Input: part model. Units: mm. Frame: model coordinates. A direction names the side the tool comes from. Round coordinates to 2 decimals unless told otherwise and drop trailing zeros. Write each loop counter-clockwise with the first axis right and the second up, starting at its lowest first coordinate (ties: lowest second). Pieces come first, ordered by that corner, then holes. Notation, with made-up numbers: (61, 51.25) -> (110, 51.25) arc R15 ccw to (110, 80.25) -> close; hole circle Ø8 at (60.25, 47). An arc over 180 degrees is marked (long way). Use CSV: the item, a comma, the result in double quotes.
```python
from build123d import *

# Parameters (mm, degrees)
SKIZZE1_W                       = 10
SKIZZE1_H                       = 46.07297751
SKIZZE1_R                       = 1.75
SKIZZE1_W_2                     = 3.5
SKIZZE1_H_2                     = 13
AUFSATZ_LINEAR_AUSTRAGEN1_DEPTH = 5
SKIZZE2_W                       = 5
SKIZZE2_H                       = 5
SCHNITT_LINEAR_AUSTRAGEN2_DEPTH = 2


with BuildPart() as part:
    # Skizze1 → Aufsatz-Linear austragen1 (new body)
    # profile 1 of 5: a face of its own
    with BuildSketch(Plane.XY):
        with Locations((0, 10.889252833)):
            Rectangle(SKIZZE1_W, SKIZZE1_H)
        with Locations((0, -1.574258412)):
            Circle(SKIZZE1_R, mode=Mode.SUBTRACT)
        with Locations((0, 7.425741588)):
            Circle(SKIZZE1_R, mode=Mode.SUBTRACT)
    # profile 2 of 5: a face of its own
    with BuildSketch(Plane.XY):
        Polygon((10, 30.925741588), (5, 30.925741588), (5, 30.675741588), (5, 18.175741588), (5, 17.925741588), (10, 17.925741588), align=None)
    # profile 3 of 5: a face of its own
    with BuildSketch(Plane.XY):
        Polygon((33.5, 17.925741588), (10, 17.925741588), (5, 17.925741588), (5, 14.925741588), (37, 14.925741588), (37, 17.925741588), align=None)
    # profile 4 of 5: a face of its own
    with BuildSketch(Plane.XY):
        Polygon((37, 33.925741588), (5, 33.925741588), (5, 30.925741588), (10, 30.925741588), (33.5, 30.925741588), (37, 30.925741588), align=None)
    # profile 5 of 5: a face of its own
    with BuildSketch(Plane.XY):
        with Locations((35.25, 24.425741588)):
            Rectangle(SKIZZE1_W_2, SKIZZE1_H_2)
    extrude(amount=AUFSATZ_LINEAR_AUSTRAGEN1_DEPTH)

    # Skizze2 → Schnitt-Linear austragen2 (cut)
    with BuildSketch(Plane(origin=(0, 0, 5), x_dir=(-1, 0, 0), z_dir=(0, 0, -1))):
        with Locations((0, 22.425741588)):
            Rectangle(SKIZZE2_W, SKIZZE2_H)
    extrude(amount=SCHNITT_LINEAR_AUSTRAGEN2_DEPTH, mode=Mode.SUBTRACT)


solid = part.part
```
Item 1: Set-up query: faces 4 (the face through (11, 16, 5)), 5 (the face through (22, 17.926, 2)), 6 (the face through (0, 19.926, 4)), 7 (the face through (5, 1, 2)), 8 (the face through (11, 16, 0)). Return all of +Z, -Z, +X, -X, +Y, -Y with unobstructed straight access to the full face (end or side cutting, diameter ignored); none if empty.
Worked answers:
face 4,"+Z, +X, -X, +Y, -Y"
face 5,"+Z, -Z"
face 6,"+Z"
face 7,"+Z, -Z, +X, -Y"
face 8,"-Z, +X, -X, +Y, -Y"
Item 2: Section query B-B on x = 0. Return the cut outline in (y, z).
Worked answers:
outline,"(-12.15, 0) -> (-3.32, 0) -> (-3.32, 5) -> (-12.15, 5) -> close; (0.18, 0) -> (5.68, 0) -> (5.68, 5) -> (0.18, 5) -> close; (9.18, 0) -> (33.93, 0) -> (33.93, 5) -> (24.93, 5) -> (24.93, 3) -> (19.93, 3) -> (19.93, 5) -> (9.18, 5) -> close"
Item 3: First-contact query: pin 1 Ø2.5 at (x, z) = (20, 1.5) entering from -Y; pin 2 Ø3 at (x, y) = (0, 7.43) entering from +Z; pin 3 Ø1.5 at (x, y) = (-0.5, 23.5) entering from +Z. Flat tips, straight axial feed; report the tip coordinate or a pass-through.
Worked answers:
pin 1,"stops at y = 14.93"
pin 2,"passes through"
pin 3,"stops at z = 3"
Item 4: Section query D-D on z = 0.95. Return the cut outline in (x, y).
Worked answers:
outline,"(-5, -12.15) -> (5, -12.15) -> (5, 14.93) -> (37, 14.93) -> (37, 33.93) -> (-5, 33.93) -> close; hole circle Ø3.5 at (0, -1.57); hole circle Ø3.5 at (0, 7.43); hole (10, 17.93) -> (33.5, 17.93) -> (33.5, 30.93) -> (10, 30.93) -> close"
Item 5: Section query A-A on y = 24. Return the cut outline in (x, z), plus the area to 3 significant figures.
Worked answers:
outline,"(-5, 0) -> (10, 0) -> (10, 5) -> (2.5, 5) -> (2.5, 3) -> (-2.5, 3) -> (-2.5, 5) -> (-5, 5) -> close; (33.5, 0) -> (37, 0) -> (37, 5) -> (33.5, 5) -> close"
area,"82.5 mm²"
Item 6: Pull-direction query (Y, two-part tool) for faces 1 (the face through (0, -12.147, 2)), 2 (the face through (37, 24, 2)), 3 (the face through (33.5, 24, 2)); classes: +Y half, -Y half, draft (parallel to the pull), parting line (faces both ways), or undercut.
Worked answers:
face 1,"-Y half"
face 2,"draft"
face 3,"undercut"
Item 7: Section query C-C on x = 27.5. Return the cut outline in (y, z), plus the area to 3 significant figures.
Worked answers:
outline,"(14.93, 0) -> (17.93, 0) -> (17.93, 5) -> (14.93, 5) -> close; (30.93, 0) -> (33.93, 0) -> (33.93, 5) -> (30.93, 5) -> close"
area,"30.0 mm²"
Item 8: Line query: line 1 (Y direction, x = 0, z = 2.9); line 2 (X direction, y = 7.5, z = 1.5); line 3 (Y direction, x = 1, z = 2.2). Output: solid intervals per line, ascending.
Worked answers:
line 1,"y = -12.15 to -3.32, 0.18 to 5.68, 9.18 to 33.93"
line 2,"x = -5 to -1.75, 1.75 to 5"
line 3,"y = -12.15 to -3.01, -0.14 to 5.99, 8.86 to 33.93"
